For this review, take the finished solid that the model builds, in its own axes (mm). Face numbers are marked on the shaded views. A direction names the side the tool comes from. Round coordinates to 2 decimals unless told otherwise and drop trailing zeros. Write each loop counter-clockwise with the first axis right and the second up, starting at its lowest first coordinate (ties: lowest second). Pieces come first, ordered by that corner, then holes. Notation, with made-up numbers: (76, -6) -> (100, -6) arc R5 cw to (100, 0) -> close; hole circle Ø5 at (23.25, -39.5). An arc over 180 degrees is marked (long way). Answer in a Markdown table with one row per item.
from build123d import *

# Parameters (mm, degrees)
SKETCH1_R               = 12
SKETCH1_R_2             = 7.5
SKETCH1_R_3             = 1.6
BOSS_EXTRUDE2_DEPTH     = 13
SKETCH1_6_W             = 50
SKETCH1_6_H             = 82
BOSS_EXTRUDE3_DEPTH     = 82
SKETCH1_5_R             = 2.85
CUT_EXTRUDE2_DEPTH      = 3.5
CUT_EXTRUDE3_DEPTH      = 14.1
CUT_EXTRUDE4_START      = -50
CUT_EXTRUDE4_DEPTH      = 14.1
CUT_EXTRUDE5_DEPTH      = 110
CUT_EXTRUDE5_DEPTH_BACK = 63
SKETCH3_W               = 62
SKETCH3_H               = 11
CUT_EXTRUDE6_DEPTH      = 1
SKETCH3_3_R             = 1.6
CUT_EXTRUDE7_DEPTH      = 14
CUT_EXTRUDE8_START      = -13
SKETCH3_5_R             = 2.85
CUT_EXTRUDE8_DEPTH      = 3.5
CUT_EXTRUDE9_START      = -13
SKETCH1_7_R             = 2.85
CUT_EXTRUDE9_DEPTH      = 3.5
CUT_EXTRUDE10_DEPTH     = 12.5
BOSS_EXTRUDE4_DEPTH     = 50
CUT_EXTRUDE11_DEPTH     = 50.5
BOSS_EXTRUDE5_DEPTH     = 20
CUT_EXTRUDE12_DEPTH     = 20
CHAMFER6_SIZE           = 10


with BuildPart() as part:
    # Sketch1 → Boss-Extrude2 (new body)
    with BuildSketch(Plane(origin=(0, 0, 0), x_dir=(0, 1, 0), z_dir=(0, 0, 1))):
        with BuildLine():
            Line((-68, -41), (-77.30151519, -41))
            Line((-77.30151519, -41), (-80, -43.69848481))
            Line((-80, -43.69848481), (-80, -80.30151519))
            Line((-80, -80.30151519), (-77.30151519, -83))
            Line((-77.30151519, -83), (-40.69848481, -83))
            Line((-40.69848481, -83), (-38, -80.30151519))
            Line((-38, -80.30151519), (-38, -71))
            Line((-38, -71), (40, -71))
            ThreePointArc((40, -71), (91, -20), (40, 31))
            Line((40, 31), (-68, 31))
            Line((-68, 31), (-68, -41))
        make_face()
        with Locations((-59, -62)):
            Circle(SKETCH1_R, mode=Mode.SUBTRACT)
        with Locations((40, -20)):
            Circle(SKETCH1_R_2, mode=Mode.SUBTRACT)
        with Locations((40, -7)):
            Circle(SKETCH1_R_3, mode=Mode.SUBTRACT)
        with Locations((49.192388155, -10.807611845)):
            Circle(SKETCH1_R_3, mode=Mode.SUBTRACT)
        with Locations((53, -20)):
            Circle(SKETCH1_R_3, mode=Mode.SUBTRACT)
        with Locations((49.192388155, -29.192388155)):
            Circle(SKETCH1_R_3, mode=Mode.SUBTRACT)
        with Locations((40, -33)):
            Circle(SKETCH1_R_3, mode=Mode.SUBTRACT)
        with Locations((30.807611845, -29.192388155)):
            Circle(SKETCH1_R_3, mode=Mode.SUBTRACT)
        with Locations((27, -20)):
            Circle(SKETCH1_R_3, mode=Mode.SUBTRACT)
        with Locations((30.807611845, -10.807611845)):
            Circle(SKETCH1_R_3, mode=Mode.SUBTRACT)
        with Locations((-74.5, -46.5)):
            Circle(SKETCH1_R_3, mode=Mode.SUBTRACT)
        with Locations((-43.5, -46.5)):
            Circle(SKETCH1_R_3, mode=Mode.SUBTRACT)
        with Locations((-43.5, -77.5)):
            Circle(SKETCH1_R_3, mode=Mode.SUBTRACT)
        with Locations((-74.5, -77.5)):
            Circle(SKETCH1_R_3, mode=Mode.SUBTRACT)
    extrude(amount=-BOSS_EXTRUDE2_DEPTH)

    # Sketch1<6> → Boss-Extrude3 (add)
    with BuildSketch(Plane(origin=(0, 0, 0), x_dir=(0, 1, 0), z_dir=(0, 0, 1))):
        with Locations((-43, 0)):
            Rectangle(SKETCH1_6_W, SKETCH1_6_H)
    extrude(amount=BOSS_EXTRUDE3_DEPTH)

    # Sketch1<5> → Cut-Extrude2 (cut)
    with BuildSketch(Plane(origin=(0, 0, 0), x_dir=(0, 1, 0), z_dir=(0, 0, 1))):
        with Locations((40, -7)):
            Circle(SKETCH1_5_R)
        with Locations((49.192388155, -10.807611845)):
            Circle(SKETCH1_5_R)
        with Locations((53, -20)):
            Circle(SKETCH1_5_R)
        with Locations((49.192388155, -29.192388155)):
            Circle(SKETCH1_5_R)
        with Locations((40, -33)):
            Circle(SKETCH1_5_R)
        with Locations((30.807611845, -29.192388155)):
            Circle(SKETCH1_5_R)
        with Locations((27, -20)):
            Circle(SKETCH1_5_R)
        with Locations((30.807611845, -10.807611845)):
            Circle(SKETCH1_5_R)
    extrude(amount=-CUT_EXTRUDE2_DEPTH, mode=Mode.SUBTRACT)

    # Sketch2 → Cut-Extrude3 (cut)
    with BuildSketch(Plane(origin=(0, -18, 0), x_dir=(-1, 0, 0), z_dir=(0, 1, 0))):
        with BuildLine():
            Line((-17.780869527, 66.393713373), (0, 78.844012252))
            Line((0, 78.844012252), (17.780869527, 66.393713373))
            ThreePointArc((17.780869527, 66.393713373), (0, 10), (-17.780869527, 66.393713373))
        make_face()
    extrude(amount=-CUT_EXTRUDE3_DEPTH, mode=Mode.SUBTRACT)

    # Sketch2<3> → Cut-Extrude4 (cut)
    with BuildSketch(Plane(origin=(0, -18, 0), x_dir=(-1, 0, 0), z_dir=(0, 1, 0)).offset(CUT_EXTRUDE4_START)):
        with BuildLine():
            Line((-17.780869527, 66.393713373), (0, 78.844012252))
            Line((0, 78.844012252), (17.780869527, 66.393713373))
            ThreePointArc((17.780869527, 66.393713373), (0, 10), (-17.780869527, 66.393713373))
        make_face()
        with BuildLine():
            Line((-12.905469818, 59.430920997), (0, 68.467428247))
            Line((0, 68.467428247), (12.905469818, 59.430920997))
            ThreePointArc((12.905469818, 59.430920997), (0, 18.5), (-12.905469818, 59.430920997))
        make_face(mode=Mode.SUBTRACT)
    extrude(amount=CUT_EXTRUDE4_DEPTH, mode=Mode.SUBTRACT)

    # Sketch2<4> → Cut-Extrude5 (cut, two sides)
    with BuildSketch(Plane(origin=(0, -18, 0), x_dir=(-1, 0, 0), z_dir=(0, 1, 0))) as cut_extrude5_sk:
        with BuildLine():
            Line((-12.905469818, 59.430920997), (0, 68.467428247))
            Line((0, 68.467428247), (12.905469818, 59.430920997))
            ThreePointArc((12.905469818, 59.430920997), (0, 18.5), (-12.905469818, 59.430920997))
        make_face()
    extrude(amount=CUT_EXTRUDE5_DEPTH, mode=Mode.SUBTRACT)
    extrude(cut_extrude5_sk.sketch, amount=-CUT_EXTRUDE5_DEPTH_BACK, mode=Mode.SUBTRACT)

    # Sketch3 → Cut-Extrude6 (cut)
    with BuildSketch(Plane.XY):
        with Locations((0, 17)):
            Rectangle(SKETCH3_W, SKETCH3_H)
    extrude(amount=-CUT_EXTRUDE6_DEPTH, mode=Mode.SUBTRACT)

    # Sketch3<3> → Cut-Extrude7 (cut, through all)
    with BuildSketch(Plane.XY):
        with Locations((-23.25, 17)):
            Circle(SKETCH3_3_R)
        with Locations((-7.75, 17)):
            Circle(SKETCH3_3_R)
        with Locations((7.75, 17)):
            Circle(SKETCH3_3_R)
        with Locations((23.25, 17)):
            Circle(SKETCH3_3_R)
    extrude(amount=-CUT_EXTRUDE7_DEPTH, mode=Mode.SUBTRACT)

    # Sketch3<5> → Cut-Extrude8 (cut)
    with BuildSketch(Plane.XY.offset(CUT_EXTRUDE8_START)):
        with Locations((-23.25, 17)):
            Circle(SKETCH3_5_R)
        with Locations((-7.75, 17)):
            Circle(SKETCH3_5_R)
        with Locations((7.75, 17)):
            Circle(SKETCH3_5_R)
        with Locations((23.25, 17)):
            Circle(SKETCH3_5_R)
    extrude(amount=CUT_EXTRUDE8_DEPTH, mode=Mode.SUBTRACT)

    # Sketch1<7> → Cut-Extrude9 (cut)
    with BuildSketch(Plane(origin=(0, 0, 0), x_dir=(0, 1, 0), z_dir=(0, 0, 1)).offset(CUT_EXTRUDE9_START)):
        with Locations((-74.5, -46.5)):
            Circle(SKETCH1_7_R)
        with Locations((-43.5, -46.5)):
            Circle(SKETCH1_7_R)
        with Locations((-43.5, -77.5)):
            Circle(SKETCH1_7_R)
        with Locations((-74.5, -77.5)):
            Circle(SKETCH1_7_R)
    extrude(amount=CUT_EXTRUDE9_DEPTH, mode=Mode.SUBTRACT)

    # Sketch4 → Cut-Extrude10 (cut)
    with BuildSketch(Plane.XZ.offset(80)):
        with BuildLine():
            Line((56, -13), (68, -13))
            ThreePointArc((68, -13), (62, -7), (56, -13))
        make_face()
    extrude(amount=-CUT_EXTRUDE10_DEPTH, mode=Mode.SUBTRACT)

    # Sketch5 → Boss-Extrude4 (add)
    with BuildSketch(Plane(origin=(0, -18, 0), x_dir=(-1, 0, 0), z_dir=(0, 1, 0))):
        Polygon((36, 0), (31, 0), (31, -5), align=None)
    extrude(amount=-BOSS_EXTRUDE4_DEPTH)

    # Sketch5<3> → Cut-Extrude11 (cut)
    with BuildSketch(Plane(origin=(0, -18, 0), x_dir=(-1, 0, 0), z_dir=(0, 1, 0))):
        Polygon((21, 82), (41, 62), (41, 82), align=None)
        Polygon((41, 5), (36, 0), (41, 0), align=None)
    extrude(amount=-CUT_EXTRUDE11_DEPTH, mode=Mode.SUBTRACT)

    # Sketch5<4> → Boss-Extrude5 (add)
    with BuildSketch(Plane(origin=(0, -18, 0), x_dir=(-1, 0, 0), z_dir=(0, 1, 0))):
        Polygon((-51, 0), (-41, 10), (-41, 0), align=None)
    extrude(amount=-BOSS_EXTRUDE5_DEPTH)

    # Sketch5<5> → Cut-Extrude12 (cut)
    with BuildSketch(Plane(origin=(0, -18, 0), x_dir=(-1, 0, 0), z_dir=(0, 1, 0))):
        Polygon((-41, 62), (-21, 82), (-41, 82), align=None)
    extrude(amount=-CUT_EXTRUDE12_DEPTH, mode=Mode.SUBTRACT)

    # Chamfer6
    chamfer6_edges = [part.edges().sort_by_distance(p)[0] for p in [
        (41, -53, 82),
    ]]
    chamfer(chamfer6_edges, length=CHAMFER6_SIZE)


solid = part.part
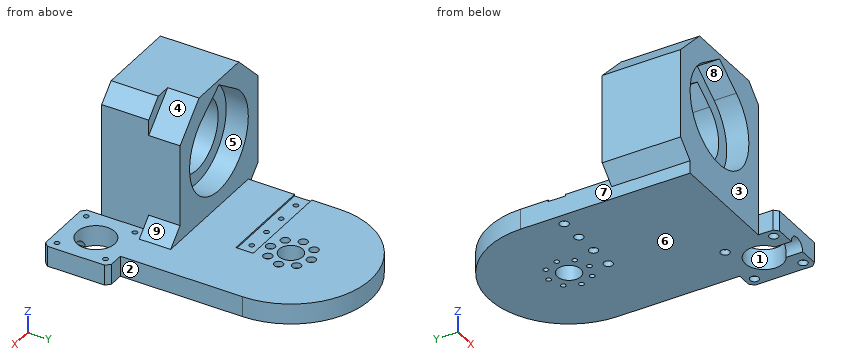
1) For the marked faces 1, 2, 3, 4 and 5, list the 3-axis set-ups (+Z, -Z, +X, -X, +Y, -Y) from which the entire face can be reached by the end or side of a thin tool; tool diameter is ignored.
Solved:
| item | result |
|---|---|
| face 1 | +Z, -Z |
| face 2 | +Z, -Z, +X, +Y |
| face 3 | +Z, -Z, -X, -Y |
| face 4 | +Z, +X, +Y |
| face 5 | +Y |
2) Consider section B-B on z = 41. State the section outline as (x, y) points.
Solved:
| item | result |
|---|---|
| outline | (-41, -68) -> (-31, -68) -> (-31, -53.9) -> (-22.5, -53.9) -> (-22.5, -32.1) -> (-31, -32.1) -> (-31, -18) -> (-41, -18) -> close; (22.5, -53.9) -> (31, -53.9) -> (31, -68) -> (41, -68) -> (41, -18) -> (31, -18) -> (31, -32.1) -> (22.5, -32.1) -> close |
3) For line 1 (Y direction, x = 77.5, z = -10.6); line 2 (Y direction, x = 23.25, z = -11.5); line 3 (Y direction, x = -23.5, z = 27), list the stretches that pass through material, from the lowest coordinate up. Write a range as [from, to].
Solved:
| item | result |
|---|---|
| line 1 | [-80, -77.35], [-71.65, -46.35], [-40.65, -38] |
| line 2 | [-68, 14.15], [19.85, 33.24], [46.76, 90.9] |
| line 3 | [-53.9, -32.1] |
4) Consider section A-A on y = -59. State the section outline as (x, z) points, then the cut area to 3 significant figures.
Solved:
| item | result |
|---|---|
| outline | (-41, 5) -> (-31, -5) -> (-31, -13) -> (50, -13) -> (50, 0) -> (41, 0) -> (41, 72) -> (31, 82) -> (-21, 82) -> (-41, 62) -> close; (74, -13) -> (83, -13) -> (83, 0) -> (74, 0) -> close; hole (-17.78, 66.39) arc R31 ccw (long way) to (17.78, 66.39) -> (0, 78.84) -> close |
| area | 4,540 mm² |
5) Mouldability with a two-part tool opening along Z and no side actions: class the marked faces 6, 7, 8 and 9 as pulls with the +Z half, pulls with the -Z half, needs draft (parallel to the pull), parting line crosses it, or undercut.
Solved:
| item | result |
|---|---|
| face 6 | pulls with the -Z half |
| face 7 | needs draft |
| face 8 | undercut |
| face 9 | pulls with the +Z half |
6) Clearance check with flat-ended pins moving along their axes: pin 1 Ø2 at (x, z) = (-26, 42.5) entering from -Y; pin 2 Ø4 at (x, z) = (23.5, 55.5) entering from +Y; pin 3 Ø8 at (x, y) = (66.5, 68) entering from +Z. State where each tip first meets the part, or that it passes through.
Solved:
| item | result |
|---|---|
| pin 1 | y = -53.9 |
| pin 2 | y = -32.1 |
| pin 3 | z = 0 |
7) Consider section C-C on z = 3. State the section outline as (x, y) points, then the cut area to 3 significant figures.
Solved:
| item | result |
|---|---|
| outline | (-39, -68) -> (41, -68) -> (41, -38) -> (48, -38) -> (48, -18) -> (-39, -18) -> close |
| area | 4,140 mm² |
